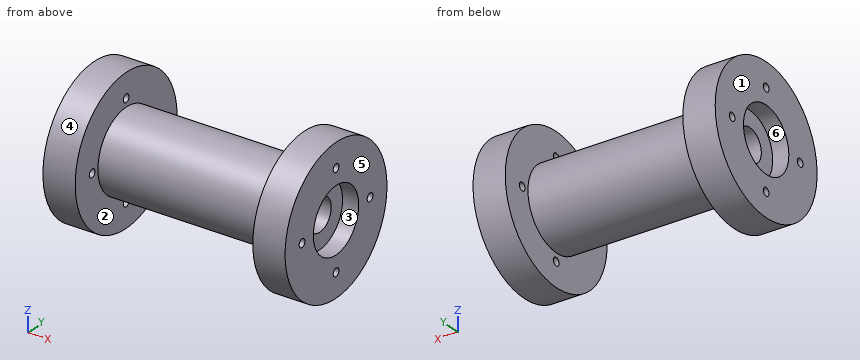
from build123d import *

# Parameters (mm, degrees)
SKETCH2_R          = 1.25
CUT_EXTRUDE1_DEPTH = 76
SKETCH3_R          = 10
CUT_EXTRUDE2_DEPTH = 5
SKETCH4_R          = 10
CUT_EXTRUDE3_DEPTH = 5


with BuildPart() as part:
    # Sketch1 → Revolve1 (revolve)
    with BuildSketch(Plane.XY):
        Polygon((0, 5), (0, 22.473684211), (10, 22.473684211), (10, 12.473684211), (65, 12.473684211), (65, 22.473684211), (75, 22.473684211), (75, 5), align=None)
    revolve(axis=Axis((0, 0, 0), (1, 0, 0)))

    # Sketch2 → Cut-Extrude1 (cut, through all)
    with BuildSketch(Plane.ZY):
        with Locations((0, 15)):
            Circle(SKETCH2_R)
        with Locations((-15, 0)):
            Circle(SKETCH2_R)
        with Locations((0, -15)):
            Circle(SKETCH2_R)
        with Locations((15, 0)):
            Circle(SKETCH2_R)
    extrude(amount=-CUT_EXTRUDE1_DEPTH, mode=Mode.SUBTRACT)

    # Sketch3 → Cut-Extrude2 (cut)
    with BuildSketch(Plane.ZY):
        Circle(SKETCH3_R)
    extrude(amount=-CUT_EXTRUDE2_DEPTH, mode=Mode.SUBTRACT)

    # Sketch4 → Cut-Extrude3 (cut)
    with BuildSketch(Plane(origin=(75, 0, 0), x_dir=(0, 0, -1), z_dir=(1, 0, 0))):
        Circle(SKETCH4_R)
    extrude(amount=-CUT_EXTRUDE3_DEPTH, mode=Mode.SUBTRACT)


solid = part.part
For this review, take the finished solid that the model builds, in its own axes (mm). Face numbers are marked on the shaded views. A direction names the side the tool comes from. Give positions to 0.01 mm unless a question says otherwise; leave off trailing zeros. Loops run counter-clockwise (first coordinate to the right, second up) from the corner with the lowest first, then second, coordinate; pieces in that order, holes last.
Item 1: Draft analysis for pull direction Y (two halves, no side actions). For the marked faces 4, 5 and 6, state which applies: +Y half, -Y half, draft (parallel to the pull), parting line (faces both ways), or undercut.
Item 2: Insertion check: pin 1 (1 mm diameter, centred on x = 67.5, z = 9.5, fed in from -Y); pin 2 (6 mm diameter, centred on x = 33.5, z = 9, fed in from -Y); pin 3 (1 mm diameter, centred on x = 59, z = -7.5, fed in from -Y). Each pin has a flat end and moves straight along its axis. Give the tip position at first contact, or say it passes through.
Item 3: For line 1 along X through (y, z) = (-18, -4.5); line 2 along Z through (x, y) = (36, 0); line 3 along Y through (x, z) = (19.5, -1.5), list the stretches that pass through material, from the lowest coordinate up.
Item 4: Take a section at C-C, the plane z = -17.5. State the section outline as (x, y) points.
Item 5: Tool access review of the marked faces 1, 2 and 3: name each direction out of +Z, -Z, +X, -X, +Y, -Y from which nothing blocks a thin tool from reaching the whole face with its end or side.
Item 6: Take a section at D-D, the plane y = -2.5. State the section outline as (x, z) points, and give its area (3 significant figures).
Item 7: Take a section at A-A, the plane z = 15. State the section outline as (x, y) points, and give its area (3 significant figures).
Calculated:
1. face 4: parting line
1. face 5: draft
1. face 6: undercut
2. pin 1: stops at y = -20.59
2. pin 2: stops at y = -10.94
2. pin 3: stops at y = -10.32
3. line 1: x = 0 to 10, 65 to 75
3. line 2: z = -12.47 to -5, 5 to 12.47
3. line 3: y = -12.38 to -4.77, 4.77 to 12.38
4. outline: (0, -14.1) - (10, -14.1) - (10, 14.1) - (0, 14.1) - close; (65, -14.1) - (75, -14.1) - (75, 14.1) - (65, 14.1) - close
5. face 1: +Z, -Z, -X, +Y, -Y
5. face 2: none
5. face 3: +X
6. outline: (0, -22.33) - (10, -22.33) - (10, -12.22) - (65, -12.22) - (65, -22.33) - (75, -22.33) - (75, -9.68) - (70, -9.68) - (70, -4.33) - (5, -4.33) - (5, -9.68) - (0, -9.68) - close; (0, 9.68) - (5, 9.68) - (5, 4.33) - (70, 4.33) - (70, 9.68) - (75, 9.68) - (75, 22.33) - (65, 22.33) - (65, 12.22) - (10, 12.22) - (10, 22.33) - (0, 22.33) - close
6. area: 1,480 mm2
7. outline: (0, -16.74) - (10, -16.74) - (10, -1.25) - (0, -1.25) - close; (0, 1.25) - (10, 1.25) - (10, 16.74) - (0, 16.74) - close; (65, -16.74) - (75, -16.74) - (75, -1.25) - (65, -1.25) - close; (65, 1.25) - (75, 1.25) - (75, 16.74) - (65, 16.74) - close
7. area: 619 mm2
